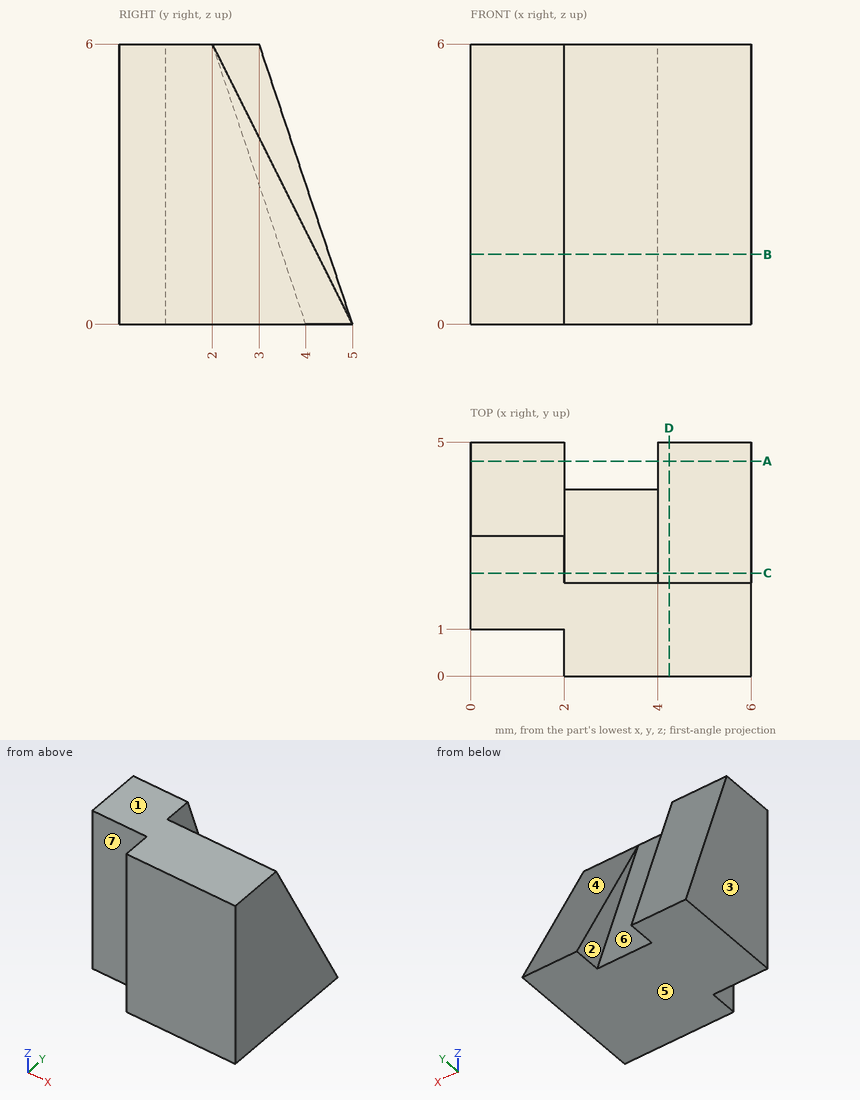
For this review, use the dimensioned drawing (mm, ordinates from the lowest corner) and the shaded views. A direction names the side the tool comes from. Give positions to 0.01 mm unless a question says otherwise; leave off trailing zeros. Order: outer loops, then holes, each group sorted by start corner. A loop starts at its lowest first (then second) coordinate and runs counter-clockwise, first axis right, second up.
1. Add section A-A, the plane y = 4.6. State the section outline as (x, z) points, then the cut area to 3 significant figures.
Solution:
outline: (0, 0) - (2, 0) - (2, 1.2) - (0, 1.2) - close; (4, 0) - (6, 0) - (6, 0.8) - (4, 0.8) - close
area: 4.00 mm2
2. For pin 1 Ø1 at (x, z) = (1, 3.5) entering from -Y; pin 2 Ø3 at (x, y) = (5.5, 4) entering from +Z; pin 3 Ø2 at (x, z) = (4, 3.5) entering from +Y, all flat-tipped, find the tip position at first contact; note any pin that passes through.
Solution:
pin 1: stops at y = 1
pin 2: stops at z = 5
pin 3: stops at y = 3.75
3. Tool access review of the marked faces 4, 5, 6 and 7: name each direction out of +Z, -Z, +X, -X, +Y, -Y from which nothing blocks a thin tool from reaching the whole face with its end or side.
Solution:
face 4: +Z, +X, +Y
face 5: -Z, +X, -X, +Y, -Y
face 6: +Z, +Y
face 7: +Z, -Z, -X, -Y
4. To check wall thickness, follow L1, parallel to X at y = 0.9, z = 3.25; L2, parallel to Y at x = 2.7, z = 2.5; L3, parallel to Y at x = 4.65, z = 0.5. State the ranges of each line that lie inside material, in increasing order.
Solution:
L1: x = 2 to 6
L2: y = 0 to 3.17
L3: y = 0 to 4.75
5. Mouldability with a two-part tool opening along X and no side actions: class the marked faces 1, 2 and 3 as +X half, -X half, draft (parallel to the pull), parting line (faces both ways), or undercut.
Solution:
face 1: draft
face 2: undercut
face 3: -X half
6. Add section C-C, the plane y = 2.2. State the section outline as (x, z) points, then the cut area to 3 significant figures.
Solution:
outline: (0, 0) - (6, 0) - (6, 5.6) - (4, 5.6) - (4, 5.4) - (2, 5.4) - (2, 6) - (0, 6) - close
area: 34.0 mm2
7. Add section B-B, the plane z = 1.5. State the section outline as (x, y) points.
Solution:
outline: (0, 1) - (2, 1) - (2, 0) - (6, 0) - (6, 4.25) - (4, 4.25) - (4, 3.5) - (2, 3.5) - (2, 4.5) - (0, 4.5) - close
8. Add section D-D, the plane x = 4.25. State the section outline as (y, z) points.
Solution:
outline: (0, 0) - (5, 0) - (2, 6) - (0, 6) - close
